For this review, take the finished solid that the model builds, in its own axes (mm). A direction names the side the tool comes from. Coordinates: 2 decimals unless noted, no trailing zeros. Loops run counter-clockwise (first coordinate to the right, second up) from the corner with the lowest first, then second, coordinate; pieces in that order, holes last. Notation, with made-up numbers: (26, 80) - (67, 80) arc R22 ccw to (67, 96) - close; hole circle Ø8 at (54.25, 6.5). An arc over 180 degrees is marked (long way). One line per item, written item: value. Start each with the question number.
1. Insertion check: pin 1 (6 mm diameter, centred on x = 16.5, y = 77.5, fed in from +Z); pin 2 (6 mm diameter, centred on x = 9.5, z = -19, fed in from -Y); pin 3 (2 mm diameter, centred on x = 24.5, z = -5, fed in from -Y). Each pin has a flat end and moves straight along its axis. Give the tip position at first contact, or say it passes through.
2. Take a section at C-C, the plane z = 38.5. State the section outline as (x, y) points.
3. Take a section at A-A, the plane y = 15.06. State the section outline as (x, z) points (3 decimals).
4. To check wall thickness, follow line 1 (Y direction, x = 24.75, z = -15) (3 decimals); line 2 (Z direction, x = 7.5, y = 13); line 3 (Z direction, x = 0.5, y = 80). State the ranges of each line that lie inside material, in increasing order. Write a range as from..to.
5. Take a section at B-B, the plane x = 25. State the section outline as (y, z) points (3 decimals), and give its area (3 significant figures).
6. Take a section at D-D, the plane x = 7.5. State the section outline as (y, z) points, and give its area (3 significant figures).
7. The part is to be moulded in two halves that separate along Y. For faces 6 (the face through (-4, 128, -14)), 7 (the face through (-21, 101, -14)), 8 (the face through (15, 85, -52)), say which applies: released by +Y, released by -Y, zero draft, split by the parting line, or undercut.
8. For faces 1 (the face through (15, 43, 0)), 2 (the face through (22.1, 21.5, -13)), 3 (the face through (-19, 100, -14)), 4 (the face through (18, 0, -27)), 5 (the face through (-17, 108, -14)), list the 3-axis set-ups (+Z, -Z, +X, -X, +Y, -Y) from which the entire face can be reached by the end or side of a thin tool; tool diameter is ignored.
Autodesk Inventor part; units mm, degrees
ref_plane "Work Plane1" through (0, 0, -15) normal (0, 0, 1) x (1, 0, 0)
ref_plane "YZ Plane" through (0, 0, 0) normal (1, 0, 0) x (0, 1, 0)
ref_plane "XZ Plane" through (0, 0, 0) normal (0, 1, 0) x (-1, 0, 0)
sketch "Sketch1" plane through (0, 0, 0) normal (0, 0, 1) x (1, 0, 0)
  line L0 (0, 0) -> (25, 0)
  line L1 (25, 0) -> (25, 40)
  line L2 (25, 40) -> (0, 40)
  line L3 (0, 40) -> (0, 0)
  dimension "d1" = 25
  dimension "d2" = 40
  dimension "d3" = 25
extrude "Extrusion1" add sketch "Sketch1" against normal blind 30
sketch "Sketch2" plane through (25, 0, 0) normal (1, 0, 0) x (0, 0, -1)
  line L0 (0, 0) -> (30, 0)
  circle A0 centre (15, 6.56) radius 2.46
extrude "Extrusion2" cut sketch "Sketch2" against normal blind 30
sketch "Sketch3" plane through (0, 0, 0) normal (-1, 0, 0) x (0, 0, 1)
  line L0 (0, 0) -> (-30, 0)
  line L1 (-25.05, 0) -> (-4.95, 0)
  line L2 (-4.95, 0) -> (-4.95, 33.12)
  line L3 (-4.95, 33.12) -> (-25.05, 33.12)
  line L4 (-25.05, 33.12) -> (-25.05, 0)
  dimension "d11" = 20.1
extrude "Extrusion3" cut sketch "Sketch3" against normal blind 20
sketch "Sketch4" plane through (0, 0, 0) normal (0, -1, 0) x (1, 0, 0)
  line L0 (20, -4.95) -> (20, -25.05)
  line L1 (20, -15) -> (25, -15)
  line L2 (25, 0) -> (25, -30)
  line L3 (20, -8.025) -> (25, -8.025)
  line L4 (25, -8.025) -> (25, -21.975)
  line L5 (25, -21.975) -> (20, -21.975)
  line L6 (20, -21.975) -> (20, -8.025)
  line L7 (20, -8.025) -> (25, -21.975) construction
  line L8 (25, -8.025) -> (20, -21.975) construction
  line L9 (25, -12.54) -> (25, -17.46)
  point P0 (0, 0)
  point P1 (22.5, -15)
  dimension "d14" = 13.95
extrude "Extrusion4" add sketch "Sketch4" along normal blind 15
sketch "Sketch5" plane through (20, 0, 0) normal (-1, 0, 0) x (0, 0, 1)
  circle A0 centre (-15, 6.56) radius 2.46
  circle A1 centre (-15, 6.56) radius 4.7025
  circle A2 centre (-15, 6.56) radius 2.46
  circle A3 centre (-15, 6.56) radius 2.46
  point P0 (0, 0)
  dimension "d17" = 9.405
extrude "Extrusion5" cut sketch "Sketch5" against normal blind 2.1
sketch "Sketch6" plane through (25, 0, 0) normal (1, 0, 0) x (0, 0, -1)
  circle A0 centre (15, 6.56) radius 4.7025
  line L0 (15, 6.56) -> (15, 23.56)
  circle A1 centre (15, 23.56) radius 2.46
  point P0 (0, 0)
  dimension "d20" = 17
  dimension "d21" = 4.92
extrude "Extrusion6" cut sketch "Sketch6" against normal blind 10 contours A1
sketch "Sketch7" plane through (20, 0, 0) normal (-1, 0, 0) x (0, 0, 1)
  circle A0 centre (-15, 23.56) radius 2.46
  circle A1 centre (-15, 23.56) radius 4.7025
  point P0 (0, 0)
  dimension "d24" = 9.405
extrude "Extrusion7" cut sketch "Sketch7" against normal blind 2.1
sketch "Sketch9" plane through (25, 0, 0) normal (1, 0, 0) x (0, 0, -1)
  circle A0 centre (15, 6.56) radius 2.46
  circle A1 centre (15, 6.56) radius 2.46
  circle A2 centre (15, 23.56) radius 2.46
  circle A3 centre (15, 23.56) radius 2.46
  line L0 (30, 40) -> (30, 0)
  line L1 (30, 0) -> (30, 40)
  line L2 (30, 40) -> (0, 40)
  line L3 (0, 40) -> (0, 0)
  line L4 (0, 0) -> (8.025, 0)
  line L5 (21.975, 0) -> (21.975, -15)
  line L6 (21.975, -15) -> (8.025, -15)
  line L7 (8.025, -15) -> (8.025, 0)
  line L8 (0, 0) -> (8.025, 0)
  line L9 (21.975, 0) -> (30, 0)
extrude "Extrusion8" add sketch "Sketch9" along normal blind 5
sketch "Sketch10" plane through (0, 40, 0) normal (0, 1, 0) x (1, 0, 0)
  line L0 (0, 30) -> (30, 30)
  line L1 (30, 0) -> (0, 0)
  line L2 (0, 30) -> (30, 30)
  line L3 (30, 30) -> (30, 0)
  line L4 (30, 0) -> (0, 0)
  line L5 (0, 0) -> (0, 30)
extrude "Extrusion9" add sketch "Sketch10" along normal blind 30
sketch "Sketch12" plane through (30, 0, 0) normal (1, 0, 0) x (0, 0, -1)
  circle A0 centre (15, 6.56) radius 2.46
  line L0 (15, 6.56) -> (15, 15.06)
  circle A1 centre (15, 15.06) radius 2.525
  point P0 (0, 0)
  dimension "d31" = 8.5
  dimension "d33" = 5.05
extrude "Extrusion10" cut sketch "Sketch12" against normal blind 30 contours A1
sketch "Sketch14" plane through (0, 0, 0) normal (0, 0, 1) x (1, 0, 0)
  line L0 (30, 70) -> (0, 70)
  line L1 (0, 70) -> (0, 85)
  line L2 (-15, 100) -> (-23, 100)
  line L3 (30, 0) -> (30, 70)
  line L4 (30, 113) -> (30, 70)
  arc A0 (0, 85) -> (-15, 100) centre (-15, 85) ccw
  line L5 (30, 105) -> (30, 100)
  line L6 (-23, 128) -> (15, 128)
  line L7 (-19, 126) -> (-23, 128)
  line L8 (-19, 126) -> (-15, 114)
  line L9 (-19, 102) -> (-23, 100)
  line L10 (-19, 102) -> (-15, 114)
  line L11 (30, 113) -> (15, 128)
  point P0 (0, 0)
  point P1 (0, 100)
  dimension "d47" = 30
  dimension "d54" = 15
  dimension "d69" = 28
extrude "Extrusion12" add sketch "Sketch14" against normal blind 30
sketch "Sketch15" plane through (0, 0, -25.05) normal (-1, 0, 0) x (0, 0, 1)
  line L0 (0, 33.12) -> (20.1, 33.12)
  line L1 (20.1, 33.12) -> (20.1, 0)
  line L2 (0, 33.12) -> (20.1, 33.12)
  line L3 (20.1, 33.12) -> (20.1, 31.1)
  line L4 (20.1, 31.1) -> (0, 31.1)
  line L5 (0, 31.1) -> (0, 33.12)
  point P0 (25.05, 0)
  dimension "d57" = 2.02
extrude "Extrusion13" add sketch "Sketch15" against normal blind 20
sketch "Sketch20" plane through (0, 0, 0) normal (0, 0, 1) x (1, 0, 0)
  arc A0 (0, 85) -> (-15, 100) centre (-15, 85) ccw
  arc A1 (0, 85) -> (-15, 100) centre (-15, 85) ccw
  line L0 (-15, 100) -> (-23, 100)
  line L1 (-15, 100) -> (-23, 100)
  line L2 (-23, 100) -> (-19, 102)
  line L3 (-23, 100) -> (-19, 102)
  line L4 (-19, 102) -> (-15, 114)
  line L5 (-19, 102) -> (-15, 114)
  line L6 (-15, 114) -> (-19, 126)
  line L7 (-15, 114) -> (-19, 126)
  line L8 (-19, 126) -> (-23, 128)
  line L9 (-19, 126) -> (-23, 128)
  line L10 (-23, 128) -> (15, 128)
  line L11 (-23, 128) -> (15, 128)
  line L12 (15, 128) -> (30, 113)
  line L13 (15, 128) -> (30, 113)
  line L14 (30, 113) -> (30, 85)
  line L15 (30, 0) -> (30, 113)
  line L16 (30, 85) -> (0, 85)
  point P0 (0, 0)
extrude "Extrusion14" add sketch "Sketch20" along normal blind 45
ref_plane "Work Plane1" through (0, 0, -15) normal (0, 0, 1) x (1, 0, 0)
mirror "Mirror1" about plane through (0, 0, -15) normal (0, 0, 1) of "Extrusion14"
properties part number "24mm_x_120mm"
Solutions:
1. pin 1: z = 0
1. pin 2: y = 31.1
1. pin 3: y = 0
2. outline: (-23, 100) - (-15, 100) arc R15 cw to (0, 85) - (30, 85) - (30, 113) - (15, 128) - (-23, 128) - (-19, 126) - (-15, 114) - (-19, 102) - close
3. outline: (0, -30) - (30, -30) - (30, -17.525) - (20, -17.525) - (20, -25.05) - (0, -25.05) - close; (0, -4.95) - (20, -4.95) - (20, -12.475) - (30, -12.475) - (30, 0) - (0, 0) - close
4. line 1: -15..4.1, 9.02..12.535, 17.585..21.1, 26.02..118.25
4. line 2: -30..-25.05, -4.95..0
4. line 3: -30..0
5. outline: (-15, -21.975) - (0, -21.975) - (0, -30) - (85, -30) - (85, -75) - (118, -75) - (118, 45) - (85, 45) - (85, 0) - (0, 0) - (0, -8.025) - (-15, -8.025) - close; hole circle Ø4.92 at (6.56, -15); hole circle Ø5.05 at (15.06, -15); hole circle Ø4.92 at (23.56, -15)
5. area: 6,660 mm2
6. outline: (0, -30) - (85, -30) - (85, -75) - (128, -75) - (128, 45) - (85, 45) - (85, 0) - (0, 0) - (0, -4.95) - (31.1, -4.95) - (31.1, -25.05) - (0, -25.05) - close
6. area: 7,080 mm2
7. face 6: released by +Y
7. face 7: undercut
7. face 8: released by -Y
8. face 1: +Z, +X, -X, -Y
8. face 2: -X
8. face 3: +Z, -Z, -X, -Y
8. face 4: -Z, +X, -X, -Y
8. face 5: +Z, -Z, -X
